Read the model definition and answer for the solid it produces. Units are mm, in the model's axes. A direction names the side the tool comes from. Round coordinates to 2 decimals unless told otherwise and drop trailing zeros. Order: outer loops, then holes, each group sorted by start corner. A loop starts at its lowest first (then second) coordinate and runs counter-clockwise, first axis right, second up. Notation, with made-up numbers: M 2.5,54 L 38.5,54 A23 ccw 38.5,62 Z; hole C 63.5,11.25 d6. An arc over 180 degrees is marked long. Use one line per item in the form item = value. Start each with the question number.
from build123d import *

# Parameters (mm, degrees)
BOSS_EXTRUDE1_DEPTH       = 4
F_4_40_TAPPED_HOLE1_D     = 2.2606
F_4_40_TAPPED_HOLE1_DEPTH = 7.6
F_4_40_TAPPED_HOLE1_TIP   = 0.679152758
F_4_40_TAPPED_HOLE2_D     = 2.2606
F_4_40_TAPPED_HOLE2_DEPTH = 7.6
F_4_40_TAPPED_HOLE2_TIP   = 0.679152758


with BuildPart() as part:
    # Sketch3 → Boss-Extrude1 (new, symmetric)
    with BuildSketch(Plane.XY):
        with BuildLine():
            Line((1, 0), (18, 0))
            Line((18, 0), (18, -4))
            Line((18, -4), (1, -4))
            ThreePointArc((1, -4), (-2.535533906, -2.535533906), (-4, 1))
            Line((-4, 1), (-4, 18))
            Line((-4, 18), (0, 18))
            Line((0, 18), (0, 1))
            ThreePointArc((0, 1), (0.292893219, 0.292893219), (1, 0))
        make_face()
    extrude(amount=BOSS_EXTRUDE1_DEPTH, both=True)

    # #4-40 Tapped Hole1
    with Locations(Plane(origin=(0, 0, 0), x_dir=(0, 0, -1), z_dir=(1, 0, 0))):
        with Locations((0, 14)):
            Hole(F_4_40_TAPPED_HOLE1_D / 2, depth=F_4_40_TAPPED_HOLE1_DEPTH)
            with Locations((0, 0, -(F_4_40_TAPPED_HOLE1_DEPTH + F_4_40_TAPPED_HOLE1_TIP / 2))):  # 118° drill point
                Cone(0, F_4_40_TAPPED_HOLE1_D / 2, F_4_40_TAPPED_HOLE1_TIP, mode=Mode.SUBTRACT)

    # #4-40 Tapped Hole2
    with Locations(Plane(origin=(0, 0, 0), x_dir=(1, 0, 0), z_dir=(0, 1, 0))):
        with Locations((14, 0)):
            Hole(F_4_40_TAPPED_HOLE2_D / 2, depth=F_4_40_TAPPED_HOLE2_DEPTH)
            with Locations((0, 0, -(F_4_40_TAPPED_HOLE2_DEPTH + F_4_40_TAPPED_HOLE2_TIP / 2))):  # 118° drill point
                Cone(0, F_4_40_TAPPED_HOLE2_D / 2, F_4_40_TAPPED_HOLE2_TIP, mode=Mode.SUBTRACT)


solid = part.part
Item 1: Section A-A (z = 0) is taken. Write down the section's boundary in (x, y), and give its area (3 significant figures).
Item 2: Find the intervals of material crossed by L1, parallel to Z at x = 14, y = -1.8; L2, parallel to Y at x = 6.25, z = 3, in increasing order. Write a range as [from, to].
Item 3: A tool of negligible diameter and unlimited length cuts with its end or side. For faces 1 (the flat face through (-0.2, 4.7, 4)), 2 (the flat face through (9, 0, 0)), from which of +Z, -Z, +X, -X, +Y, -Y can it reach the whole face along a straight path? Write none if from no direction.
Item 4: Section B-B (y = 14) is taken. Write down the section's boundary in (x, z), and give its area (3 significant figures).
Item 5: For a pull along Y with two mould halves and no side action, classify faces 3 (the cylindrical face through (-2.028, 12.897, -0.245)), 4 (the cylindrical face through (15.13, -2.03, -0.05)), 5 (the flat face through (10, -4, 0)), 6 (the cylindrical face through (0.285, 0.301, 0.056)) as pulls with the +Y half, pulls with the -Y half, needs draft (parallel to the pull), parting line crosses it, or undercut.
Item 6: Given P1, Ø2, axis at x = 14, z = 0, coming from the -Y side; P2, Ø4, axis at x = 8, z = 1, coming from the +Y side; P3, Ø4, axis at y = 3, z = -1.5, coming from the +X side, each flat-ended and moving along its own axis, determine where each tip first touches the part or whether it passes through.
Item 7: Section D-D (z = -1.5) is taken. Write down the section's boundary in (x, y).
The answers:
q1.outline = M -4,1 A5 ccw 1,-4 L 12.87,-4 L 12.87,0 L 1,0 A1 cw 0,1 L 0,12.87 L -4,12.87 Z; M -4,15.13 L 0,15.13 L 0,18 L -4,18 Z; M 15.13,-4 L 18,-4 L 18,0 L 15.13,0 Z
q1.area = 137 mm²
q2.L1 = [-4, -1.13], [1.13, 4]
q2.L2 = [-4, 0]
q3.face_1 = +Z, +X, -X, +Y, -Y
q3.face_2 = +Z, -Z, +X, +Y
q4.outline = M -4,-4 L 0,-4 L 0,-1.13 L -4,-1.13 Z; M -4,1.13 L 0,1.13 L 0,4 L -4,4 Z
q4.area = 23.0 mm²
q5.face_3 = undercut
q5.face_4 = needs draft
q5.face_5 = pulls with the -Y half
q5.face_6 = pulls with the +Y half
q6.P1 = through
q6.P2 = 0
q6.P3 = 0
q7.outline = M -4,1 A5 ccw 1,-4 L 18,-4 L 18,0 L 1,0 A1 cw 0,1 L 0,18 L -4,18 Z
